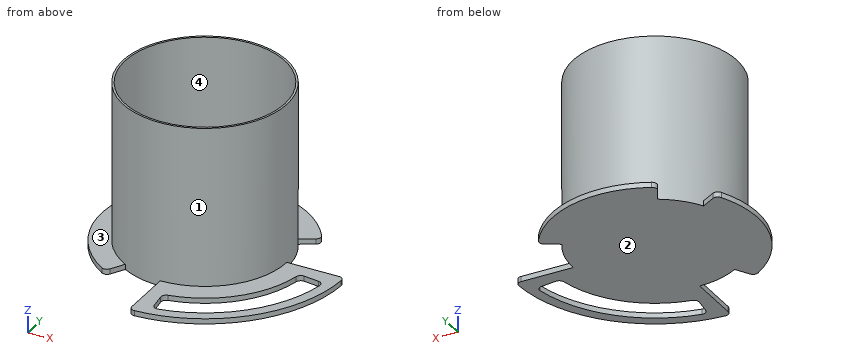
from build123d import *

# Parameters (mm, degrees)
SKETCH_R           = 78.5
SKETCH_R_2         = 76.5
PAD_DEPTH          = 153
SKETCH001_R        = 78.5
PAD001_DEPTH       = 5
PAD002_DEPTH       = 5
POLARPATTERN_COUNT = 3
PAD003_DEPTH       = 5


with BuildPart() as part:
    # Sketch → Pad (new body)
    with BuildSketch(Plane.XY):
        Circle(SKETCH_R)
        Circle(SKETCH_R_2, mode=Mode.SUBTRACT)
    extrude(amount=PAD_DEPTH)

    # Sketch001 (on Face3 of Pad) → Pad001 (join)
    with BuildSketch(Plane(origin=(0, 0, 0), x_dir=(1, 0, 0), z_dir=(0, 0, -1))):
        Circle(SKETCH001_R)
    extrude(amount=PAD001_DEPTH)

    # Sketch002 (on Face5 of Pad001) → Pad002 (join)
    with BuildSketch(Plane(origin=(0, 0, -5), x_dir=(1, 0, 0), z_dir=(0, 0, -1))):
        with BuildLine():
            ThreePointArc((78.5, 0), (55.507882, 55.507882), (0, 78.5))
            Line((0, 78.5), (0, 93.366214))
            ThreePointArc((5.26738, 98.35906), (1.560298, 96.99505), (0, 93.366214))
            ThreePointArc((98.35906, 5.26738), (69.650018, 69.650018), (5.26738, 98.35906))
            ThreePointArc((93.366214, 0), (96.99505, 1.560298), (98.35906, 5.26738))
            Line((78.5, 0), (93.366214, 0))
        make_face()
    pad002 = extrude(amount=-PAD002_DEPTH)

    # PolarPattern: Pad002 ×3 about axis
    polarpattern_axis = Axis((0, 0, -5), (0, 0, -1))
    for i in range(1, POLARPATTERN_COUNT):
        add(pad002.rotate(polarpattern_axis, i * 360 / POLARPATTERN_COUNT))

    # Sketch003 (on Face23 of PolarPattern) → Pad003 (join)
    with BuildSketch(Plane(origin=(0, 0, -5), x_dir=(1, 0, 0), z_dir=(0, 0, -1))):
        with BuildLine():
            ThreePointArc((133.3989, 5.194553), (94.398755, 94.398755), (5.194553, 133.3989))
            ThreePointArc((5.194553, 133.3989), (1.533933, 132.006349), (0, 128.402687))
            Line((0, 0), (0, 128.402687))
            Line((0, 0), (128.402687, 0))
            ThreePointArc((128.402687, 0), (132.006349, 1.533933), (133.3989, 5.194553))
        make_face()
        with BuildLine():
            ThreePointArc((121.654228, 21.272019), (87.327687, 87.327687), (21.272019, 121.654228))
            ThreePointArc((21.272019, 121.654228), (17.45138, 120.759069), (15.453579, 117.381587))
            Line((13.493688, 102.494733), (15.453579, 117.381587))
            ThreePointArc((13.493688, 102.494733), (14.41176, 98.895028), (17.559564, 96.922194))
            ThreePointArc((96.922194, 17.559564), (69.650018, 69.650018), (17.559564, 96.922194))
            ThreePointArc((96.922194, 17.559564), (98.895028, 14.41176), (102.494733, 13.493688))
            Line((102.494733, 13.493688), (117.381587, 15.453579))
            ThreePointArc((117.381587, 15.453579), (120.759069, 17.45138), (121.654228, 21.272019))
        make_face(mode=Mode.SUBTRACT)
    extrude(amount=-PAD003_DEPTH)


solid = part.part
Model file for the job. Use its own axes, mm. Face numbers are marked on the shaded views. A direction names the side the tool comes from. Coordinates: 2 decimals unless noted, no trailing zeros. Write each loop counter-clockwise with the first axis right and the second up, starting at its lowest first coordinate (ties: lowest second). Pieces come first, ordered by that corner, then holes. Notation, with made-up numbers: (7, 54) -> (35, 54) arc R33 cw to (35, 89) -> close; hole circle Ø2 at (-28, 76.5). An arc over 180 degrees is marked (long way). One line per item, written item: value. Start each with the question number.
1) Pull direction Y, two halves, no side cores. Call the marked faces 3 and 4: +Y half, -Y half, draft (parallel to the pull), parting line (faces both ways), or undercut.
2) Which spindle directions (+Z, -Z, +X, -X, +Y, -Y) get a long thin tool onto all of the face, cutting with end or side? Do the marked faces 1 and 2. Say none if no direction does.
3) Slice it at A-A on y = -93. Write the cut outline in (x, z), then the cut area to 3 significant figures.
4) Probe probe 1 along Y at (x, z) = (0, 69); probe 2 along Z at (x, y) = (39.5, -72). List the from-to ranges inside material, lowest first.
5) Slice it at D-D on x = -35. Write the cut outline in (y, z), then the cut area to 3 significant figures.
6) Slice it at C-C on z = 79. Write the cut outline in (x, y).
7) Slice it at B-B on x = 110.5. Write the cut outline in (y, z).
8) Flat gauge pins, fed straight in: pin 1 Ø18 at (x, y) = (-58, -5.5) entering from +Z; pin 2 Ø5 at (y, z) = (10, 109) entering from -X; pin 3 Ø5.5 at (y, z) = (-112, -3.5) entering from -X; pin 4 Ø6 at (x, y) = (23.5, -99) entering from -Z. Where does each tip first touch, or does it go through?
Answers follow:
1. face 3: draft
1. face 4: undercut
2. face 1: +Z
2. face 2: -Z, +X, -X, +Y, -Y
3. outline: (0, -5) -> (32.45, -5) -> (32.45, 0) -> (0, 0) -> close; (81.26, -5) -> (95.78, -5) -> (95.78, 0) -> (81.26, 0) -> close
3. area: 235 mm2
4. probe 1: -78.5 to -76.5, 76.5 to 78.5
4. probe 2: -5 to 0
5. outline: (-70.27, -5) -> (92.07, -5) -> (92.07, 0) -> (70.27, 0) -> (70.27, 153) -> (68.02, 153) -> (68.02, 0) -> (-68.02, 0) -> (-68.02, 153) -> (-70.27, 153) -> close
5. area: 1,500 mm2
6. outline: circle Ø157 at (0, 0); hole circle Ø153 at (0, 0)
7. outline: (-74.91, -5) -> (-55.15, -5) -> (-55.15, 0) -> (-74.91, 0) -> close; (-14.55, -5) -> (0, -5) -> (0, 0) -> (-14.55, 0) -> close
8. pin 1: z = 0
8. pin 2: x = -78.14
8. pin 3: x = 0
8. pin 4: through
